```python
from build123d import *

# Parameters (mm, degrees)
SKETCH1_R          = 17.5
SKETCH1_R_2        = 2.5
BODY_DEPTH         = 2
SKETCH4_R          = 3.45
SKETCH4_R_2        = 2.5
SHAFT_DEPTH        = 13
SKETCH5_R          = 17.5
SKETCH5_R_2        = 16.5
BORDER_DEPTH       = 8
SKETCH3_R          = 1.6
SCREW_HOLES_DEPTH  = 3
SCREW_CHAMFER_SIZE = 1


with BuildPart() as part:
    # Sketch1 → Body (new body)
    with BuildSketch(Plane(origin=(0, 0, 0), x_dir=(1, 0, 0), z_dir=(0, 1, 0))):
        with Locations(Location((0, 0, 0), (0, 0, 270))):
            Circle(SKETCH1_R)
        with Locations(Location((0, 0, 0), (0, 0, 270))):
            Circle(SKETCH1_R_2, mode=Mode.SUBTRACT)
    extrude(amount=BODY_DEPTH)

    # Sketch4 → Shaft (add)
    with BuildSketch(Plane(origin=(0, 2, 0), x_dir=(1, 0, 0), z_dir=(0, 1, 0))):
        with Locations(Location((0, 0, 0), (0, 0, 270))):
            Circle(SKETCH4_R)
        with Locations(Location((0, 0, 0), (0, 0, 270))):
            Circle(SKETCH4_R_2, mode=Mode.SUBTRACT)
    extrude(amount=SHAFT_DEPTH)

    # Sketch5 → Border (add)
    with BuildSketch(Plane(origin=(0, 2, 0), x_dir=(1, 0, 0), z_dir=(0, 1, 0))):
        with Locations(Location((0, 0, 0), (0, 0, 270))):
            Circle(SKETCH5_R)
        with Locations(Location((0, 0, 0), (0, 0, 270))):
            Circle(SKETCH5_R_2, mode=Mode.SUBTRACT)
    extrude(amount=BORDER_DEPTH)

    # Sketch3 → Screw holes (cut)
    with BuildSketch(Plane(origin=(0, 0, 0), x_dir=(-1, 0, 0), z_dir=(0, -1, 0))):
        with Locations(Location((5.656854249, 5.656854249, 0), (0, 0, 90))):
            Circle(SKETCH3_R)
        with Locations(Location((5.656854249, -5.656854249, 0), (0, 0, 90))):
            Circle(SKETCH3_R)
        with Locations(Location((-5.656854249, -5.656854249, 0), (0, 0, 90))):
            Circle(SKETCH3_R)
        with Locations(Location((-5.656854249, 5.656854249, 0), (0, 0, 90))):
            Circle(SKETCH3_R)
    extrude(amount=-SCREW_HOLES_DEPTH, mode=Mode.SUBTRACT)

    # Screw chamfer
    screw_chamfer_edges = [part.edges().sort_by_distance(p)[0] for p in [
        (0, 0, -17.5),
    ]]
    chamfer(screw_chamfer_edges, length=SCREW_CHAMFER_SIZE)


solid = part.part
```
Could you check a few things on this model? Use its own coordinates, in mm. A direction names the side the tool comes from. Round coordinates to 2 decimals unless told otherwise and drop trailing zeros. Write each loop counter-clockwise with the first axis right and the second up, starting at its lowest first coordinate (ties: lowest second). Pieces come first, ordered by that corner, then holes. Notation, with made-up numbers: M 81,-18 L 127,-18 A11 ccw 127,1 Z; hole C -31,42.5 d10. An arc over 180 degrees is marked long. Answer in a Markdown table with one row per item. Add a question column.
Q1. Imagine slicing it at C-C (y = 8). Please give me the cut outline in (x, z).
Q2. Imagine slicing it at D-D (x = 5). Give the number of separate pieces and of enclosed holes in the cut face, then the cut area to 3 significant figures.
Q3. Imagine slicing it at B-B (z = 0). Please give me the cut outline in (x, y), then the cut area to 3 significant figures.
Q4. Imagine slicing it at A-A (x = 0). Please give me the cut outline in (y, z), then the cut area to 3 significant figures.
Q5. Will these pins go through, and if not, where does the flat tip stop? pin 1 Ø1.9 at (x, z) = (-5.66, 5.66) entering from +Y; pin 2 Ø6 at (x, y) = (-11, 10) entering from +Z; pin 3 Ø12 at (x, z) = (14, 1) entering from +Y.
Q6. On a 3-axis mill with a long thin cutter (end or side, diameter ignored), from which of +Z, -Z, +X, -X, +Y, -Y can I reach the whole of each face in a straight line? I mean faces 1 (the cylindrical face through (-16.108, 5.944, -3.577)), 2 (the cylindrical face through (-2.44, 7.4, -0.54)). Say none if no direction works.
Q7. If we mould it in two halves opening along X, with no side actions, what happens to faces 3 (the flat face through (-3, 0, 0)), 4 (the cylindrical face through (-10.648, 5.437, -13.887)), 5 (the cylindrical face through (-7.076, 0.986, 4.919))? For each: +X half, -X half, draft (parallel to the pull), parting line (faces both ways), or undercut.
Q8. If I drill on line 1 (X direction, y = 5.25, z = -0.5); line 2 (Y direction, x = 8.5, z = -8.5); line 3 (X direction, y = 3.5, z = 1.5), over which ranges is the centre line in solid material (lowest first)? Write a range as from..to.
Values:
| question | item | result |
|---|---|---|
| 1 | outline | C 0,0 d35; C 0,0 d6.9; hole C 0,0 d33; hole C 0,0 d5 |
| 2 | separate pieces | 3 |
| 2 | enclosed holes | 0 |
| 2 | area | 71.1 mm^2 |
| 3 | outline | M -17.5,1 L -16.5,0 L -2.5,0 L -2.5,15 L -3.45,15 L -3.45,2 L -16.5,2 L -16.5,10 L -17.5,10 Z; M 2.5,0 L 16.5,0 L 17.5,1 L 17.5,10 L 16.5,10 L 16.5,2 L 3.45,2 L 3.45,15 L 2.5,15 Z |
| 3 | area | 99.7 mm^2 |
| 4 | outline | M 0,-16.5 L 1,-17.5 L 10,-17.5 L 10,-16.5 L 2,-16.5 L 2,-3.45 L 15,-3.45 L 15,-2.5 L 0,-2.5 Z; M 0,2.5 L 15,2.5 L 15,3.45 L 2,3.45 L 2,16.5 L 10,16.5 L 10,17.5 L 1,17.5 L 0,16.5 Z |
| 4 | area | 99.7 mm^2 |
| 5 | pin 1 | through |
| 5 | pin 2 | z = 15.56 |
| 5 | pin 3 | y = 10 |
| 6 | face 1 | +Y |
| 6 | face 2 | +Y, -Y |
| 7 | face 3 | draft |
| 7 | face 4 | parting line |
| 7 | face 5 | undercut |
| 8 | line 1 | -17.49..-16.49, -3.41..-2.45, 2.45..3.41, 16.49..17.49 |
| 8 | line 2 | 0..2 |
| 8 | line 3 | -17.44..-16.43, -3.11..-2, 2..3.11, 16.43..17.44 |
